Input: part model. Units: mm. Frame: model coordinates. Face numbers are marked on the shaded views. Coordinates: 2 decimals unless noted, no trailing zeros. Order: outer loops, then holes, each group sorted by start corner. A loop starts at its lowest first (then second) coordinate and runs counter-clockwise, first axis right, second up. Notation, with made-up numbers: M 14,48.25 L 23,48.25 A22 cw 23,58.25 Z; hole C 26.5,17 d3. An arc over 180 degrees is marked long. One line per item, written item: value.
```python
from build123d import *

# Parameters (mm, degrees)
ESBO_O1_W                = 37
ESBO_O1_H                = 22.5
RESSALTO_EXTRUS_O1_DEPTH = 1
ESBO_O2_R                = 2.25
ESBO_O2_R_2              = 3.5
CORTE_EXTRUS_O1_DEPTH    = 1
ESBO_O3_W                = 37
ESBO_O3_H                = 7
RESSALTO_EXTRUS_O2_DEPTH = 1
ESBO_O5_R                = 1.5
CORTE_EXTRUS_O2_DEPTH    = 1


with BuildPart() as part:
    # Esboço1 → Ressalto-extrusão1 (new body)
    with BuildSketch(Plane.XY):
        with Locations((18.5, 11.25)):
            Rectangle(ESBO_O1_W, ESBO_O1_H)
    extrude(amount=RESSALTO_EXTRUS_O1_DEPTH)

    # Esboço2 → Corte-extrusão1 (cut)
    with BuildSketch(Plane.XY.offset(1)):
        with Locations((5.5, 19.74)):
            Circle(ESBO_O2_R)
        with Locations((25, 11.25)):
            Circle(ESBO_O2_R_2)
        with Locations(Location((5.5, 2.76, 0), (0, 0, 180))):
            Circle(ESBO_O2_R)
        with Locations(Location((12, 11.25, 0), (0, 0, 180))):
            Circle(ESBO_O2_R_2)
        with Locations((31.5, 2.76)):
            Circle(ESBO_O2_R)
        with Locations(Location((31.5, 19.74, 0), (0, 0, 180))):
            Circle(ESBO_O2_R)
    extrude(amount=-CORTE_EXTRUS_O1_DEPTH, mode=Mode.SUBTRACT)

    # Esboço3 → Ressalto-extrusão2 (add)
    with BuildSketch(Plane(origin=(0, 22.5, 0), x_dir=(1, 0, 0), z_dir=(0, 1, 0))):
        with Locations((18.5, -3.5)):
            Rectangle(ESBO_O3_W, ESBO_O3_H)
    extrude(amount=RESSALTO_EXTRUS_O2_DEPTH)

    # Esboço5 → Corte-extrusão2 (cut)
    with BuildSketch(Plane(origin=(0, 23.5, 0), x_dir=(1, 0, 0), z_dir=(0, 1, 0))):
        with Locations(Location((1.8, -3.5, 0), (0, 0, 270))):
            Circle(ESBO_O5_R)
        with Locations(Location((10, -3.5, 0), (0, 0, 270))):
            Circle(ESBO_O5_R)
        with Locations(Location((15, -3.5, 0), (0, 0, 270))):
            Circle(ESBO_O5_R)
        with Locations(Location((22, -3.5, 0), (0, 0, 270))):
            Circle(ESBO_O5_R)
        with Locations(Location((27, -3.5, 0), (0, 0, 270))):
            Circle(ESBO_O5_R)
        with Locations(Location((35.2, -3.5, 0), (0, 0, 270))):
            Circle(ESBO_O5_R)
    extrude(amount=-CORTE_EXTRUS_O2_DEPTH, mode=Mode.SUBTRACT)


solid = part.part
```
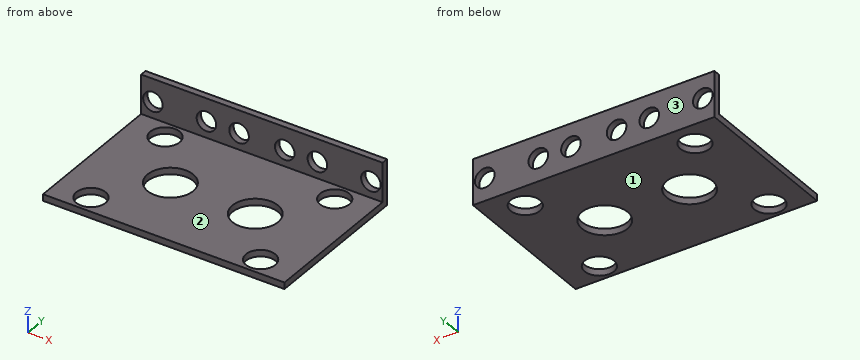
(1) Cut plane D-D on z = 3.25. Output: boundary loops of the cut face in (x, y).
Data:
outline: M 0,22.5 L 0.32,22.5 L 0.32,23.5 L 0,23.5 Z; M 3.28,22.5 L 8.52,22.5 L 8.52,23.5 L 3.28,23.5 Z; M 11.48,22.5 L 13.52,22.5 L 13.52,23.5 L 11.48,23.5 Z; M 16.48,22.5 L 20.52,22.5 L 20.52,23.5 L 16.48,23.5 Z; M 23.48,22.5 L 25.52,22.5 L 25.52,23.5 L 23.48,23.5 Z; M 28.48,22.5 L 33.72,22.5 L 33.72,23.5 L 28.48,23.5 Z; M 36.68,22.5 L 37,22.5 L 37,23.5 L 36.68,23.5 Z
(2) Cut plane C-C on x = 31.5. Output: boundary loops of the cut face in (y, z), plus the area to 3 significant figures.
Data:
outline: M 0,0 L 0.51,0 L 0.51,1 L 0,1 Z; M 5.01,0 L 17.49,0 L 17.49,1 L 5.01,1 Z; M 21.99,0 L 23.5,0 L 23.5,7 L 22.5,7 L 22.5,1 L 21.99,1 Z
area: 20.5 mm2
(3) Ray query, line 1 (Y direction, x = 5.5, z = 0.35); line 2 (X direction, y = 11, z = 0.75); line 3 (Z direction, x = 28.5, y = 8.75). Return the intervals inside material, ascending. Write a range as from..to.
Data:
line 1: y = 0..0.51, 5.01..17.49, 21.99..23.5
line 2: x = 0..8.51, 15.49..21.51, 28.49..37
line 3: z = 0..1
(4) Draft query along Z for the marked faces 1, 2 and 3. Return one class per face: released by +Z, released by -Z, zero draft, split by the parting line, or undercut.
Data:
face 1: released by -Z
face 2: released by +Z
face 3: zero draft
(5) First-contact query: pin 1 (4 mm diameter, centred on x = 15, z = 3.5, fed in from -Y); pin 2 (8 mm diameter, centred on x = 12, y = 11.25, fed in from +Z). Flat tips, straight axial feed; report the tip coordinate or a pass-through.
Data:
pin 1: stops at y = 22.5
pin 2: stops at z = 1
(6) Cut plane B-B on x = 25. Output: boundary loops of the cut face in (y, z).
Data:
outline: M 0,0 L 7.75,0 L 7.75,1 L 0,1 Z; M 14.75,0 L 23.5,0 L 23.5,7 L 22.5,7 L 22.5,1 L 14.75,1 Z
(7) Cut plane A-A on y = 2.76. Output: boundary loops of the cut face in (x, z).
Data:
outline: M 0,0 L 3.25,0 L 3.25,1 L 0,1 Z; M 7.75,0 L 29.25,0 L 29.25,1 L 7.75,1 Z; M 33.75,0 L 37,0 L 37,1 L 33.75,1 Z
